For this review, take the finished solid that the model builds, in its own axes (mm). A direction names the side the tool comes from. Coordinates: 2 decimals unless noted, no trailing zeros. Loops run counter-clockwise (first coordinate to the right, second up) from the corner with the lowest first, then second, coordinate; pieces in that order, holes last.
1. To check wall thickness, follow probe 1 along X at (y, z) = (1.5, -0.6); probe 2 along Z at (x, y) = (-0.5, -0.1); probe 3 along Y at (x, z) = (-0.25, -0.35). State the ranges of each line that lie inside material, in increasing order.
2. Take a section at B-B, the plane x = -1. State the section outline as (y, z) points, then the cut area to 3 significant figures.
3. Take a section at A-A, the plane x = 4.25. State the section outline as (y, z) points, then the cut area to 3 significant figures.
4. Mouldability with a two-part tool opening along Y and no side actions: class faces 4 (the face through (-1.09, 0.51, 0.86)), 5 (the face through (2.86, -1.5, -0.07)), 6 (the face through (6, 0, 0)) as pulls with the +Y half, pulls with the -Y half, needs draft (parallel to the pull), parting line crosses it, or undercut.
5. Clearance check with flat-ended pins moving along their axes: P1, Ø0.9, axis at x = -1, z = 0.5, coming from the -Y side; P2, Ø3, axis at y = -1.5, z = 0.5, coming from the +X side; P3, Ø1.5, axis at x = 2, y = 0.5, coming from the +Z side. State where each tip first meets the part, or that it passes through.
6. Machinability: for faces 1 (the face through (-0.193, -2.262, 1.734)), 2 (the face through (0, 0, -2)), 3 (the face through (-1, 1, 0)), which of the approach directions +Z, -Z, +X, -X, +Y, -Y give a long, thin tool a straight path to every point of the face, cutting with its end or side? Answer none if there is none.
Autodesk Inventor part; units mm, degrees
ref_plane "Work Plane1" through (30, 0, 0) normal (0, -0.5, 0.866) x (1, 0, 0)
ref_plane "YZ Plane" through (0, 0, 0) normal (1, 0, 0) x (0, 1, 0)
ref_plane "XZ Plane" through (0, 0, 0) normal (0, 1, 0) x (-1, 0, 0)
sketch "Sketch1" plane through (0, 0, 0) normal (0, 0, 1) x (1, 0, 0)
  line L0 (0.0567, 0) -> (6, 0)
  line L1 (6, 0) -> (6, 1.5)
  line L2 (6, 1.5) -> (1, 1.5)
  line L3 (1, 1.5) -> (0.6933, 1.5)
  line L4 (0.6933, 1.5) -> (0, 1.5)
  line L5 (0, 1.5) -> (0, 2.85)
  line L6 (0, 2.85) -> (-1.65, 2.85)
  line L7 (-1.65, 2.85) -> (-1.65, 1.1547)
  line L8 (-1.65, 1.1547) -> (-0.61, 1.1547)
  line L9 (-0.61, 1.1547) -> (0.0567, 0)
  line L10 (-3.18, 0) -> (7.53, 0)
  line L11 (0, -0.57) -> (0, 3.42)
  line L12 (1, 1.5) -> (0, 1.5) construction
  dimension "d0" = 5
  dimension "d1" = 0.3067
  dimension "d2" = 1.65
  dimension "d3" = 1.04
  dimension "d4" = 60
  dimension "d5" = 3
  dimension "d6" = 3
  dimension "d7" = 2.3094
  dimension "d8" = 5.7
  dimension "d19" = 6
revolve "Body" add sketch "Sketch1" angle 360 about axis through (0.0567, 0, 0) along (1, 0, 0) contours L9 L11 L4 L3 L2 L1 L0 | L9 L8 L7 L6 L5 L11
sketch "Sketch2" plane through (-1.65, 0, 0) normal (-1, 0, 0) x (0, 0, 1)
  circle A0 centre (0, 0) radius 1.1547
  line L0 (0, -3.99) -> (0, 3.99)
  line L1 (-3.99, 0) -> (3.99, 0)
  line L2 (1.1547, 0) -> (0.5774, -1)
  line L3 (0.5774, -1) -> (-0.5774, -1)
  line L4 (-0.5774, -1) -> (-1.1547, 0)
  line L5 (-1.1547, 0) -> (-0.5774, 1)
  line L6 (-0.5774, 1) -> (0.5774, 1)
  line L7 (0.5774, 1) -> (1.1547, 0)
extrude "Slot" add sketch "Sketch2" against normal up to next contours L7 A0 | A0 L2 | L6 L0 A0 | A0 L0 L3 | L0 L6 A0 | A0 L3 L0 | L4 A0 | A0 L5
fillet "Fillet1" radius 1.27 1 edges at (-1.65, -2.85, 0)
thread "Thread"
chamfer "Chamfer1" distance 0.3067 distance2 0.3067 1 edges at (6, -1.5, 0) measured on face at (6, -0.2617, -0.7882)
fillet "Fillet2" radius 0.1 1 edges at (0, -1.5, 0)
ref_plane "Work Plane1" through (30, 0, 0) normal (0, -0.5, 0.866) x (1, 0, 0)
equation "\"d0\" = GEL"
equation "\"d1\" = GAL"
equation "\"d2\" = KOH"
equation "\"d3\" = INTI"
equation "\"d5\" = GD"
equation "\"d6\" = BDM"
equation "\"d7\" = 1.1547 * SW"
equation "\"d8\" = KOD"
equation "\"d19\" = NLG"
equation "\"d16\" = RR"
equation "\"d12\" = GEL"
equation "\"d14\" = -0.5 * SPD + 0.5 * GD"
equation "\"d15\" = GUL"
equation "\"d29\" = R"
equation "\"GD\" = NND"
equation "\"NLG\" = 6"
equation "\"GEL\" = 5"
equation "\"KOD\" = 5.7"
equation "\"KOH\" = 1.65"
equation "\"INTI\" = 1.04"
equation "\"GAL\" = 0.61345 * PTC"
equation "\"GUL\" = 0.61345 * PTC"
equation "\"BDM\" = NND"
equation "\"SW\" = 2"
equation "\"RR\" = 1.27"
equation "\"SPD\" = 2.38655"
equation "\"d28\" = R"
equation "\"R\" = 0.1"
equation "\"TOA\" = 30deg"
equation "\"THREADDIA\" = 3"
equation "\"KOD1\" = KOD - 2 * RR"
equation "\"PTC\" = 0.5"
equation "\"NND\" = 3"
equation "\"E0\" = 1.155 * SW"
equation "\"GD1\" = THREADDIA - 1.2269 * PTC"
properties part number "ANSI B18.3.4M - M3 x 0.5 x 6, FHSBHCSM" material "Steel, Mild"
Results list:
1. probe 1: x = -1.65 to 0
1. probe 2: z = -2.84 to -0.96, 0.96 to 2.84
1. probe 3: y = -2.83 to -0.4, 0.4 to 2.83
2. outline: circle Ø5.38 at (0, 0); hole (-1, -0.58) - (0, -1.15) - (1, -0.58) - (1, 0.58) - (0, 1.15) - (-1, 0.58) - close
2. area: 19.2 mm2
3. outline: circle Ø3 at (0, 0)
3. area: 7.07 mm2
4. face 4: undercut
4. face 5: parting line crosses it
4. face 6: needs draft
5. P1: stops at y = -2.82
5. P2: stops at x = 6
5. P3: stops at z = 1.5
6. face 1: +X, -X
6. face 2: +X
6. face 3: -X
